from build123d import *

# Parameters (mm, degrees)
F0_R      = 2.05
F1_DEPTH  = 0.8
F2_DEPTH  = 19.2
F3_R      = 4.55
F4_DEPTH  = 2.1
F5_DEPTH  = 4
F6_DEPTH  = 10.3
F8_W      = 14.5
F8_H      = 16.5
F12_DEPTH = 0.65
F13_R     = 2.1
F14_SIZE  = 0.2


with BuildPart() as f1:
    # F0 (on Top) → F1 (new body)
    with BuildSketch(Plane.XY):
        with BuildLine():
            ThreePointArc((-13.5296202829, -3.5), (-13.975, 0), (-13.5296202829, 3.5))
            Line((-13.5296202829, 3.5), (-17.45, 3.5))
            ThreePointArc((-17.45, 3.5), (-20.95, 0), (-17.45, -3.5))
            Line((-17.45, -3.5), (-13.5296202829, -3.5))
        make_face()
        with Locations((-17.45, 0)):
            Circle(F0_R, mode=Mode.SUBTRACT)
    extrude(amount=F1_DEPTH)



with BuildPart() as f1b:
    # F0 (on Top) → F1, piece 2 (new body)
    with BuildSketch(Plane.XY):
        with BuildLine():
            Line((17.45, 3.5), (13.5296202829, 3.5))
            ThreePointArc((13.5296202829, 3.5), (13.975, 0), (13.5296202829, -3.5))
            Line((13.5296202829, -3.5), (17.45, -3.5))
            ThreePointArc((17.45, -3.5), (20.95, 0), (17.45, 3.5))
        make_face()
        with Locations((17.45, 0)):
            Circle(F0_R, mode=Mode.SUBTRACT)
    extrude(amount=F1_DEPTH)


with BuildPart() as f1_1:
    add(f1.part)

    add(f1b.part)  # F2 merges F1b
    # F0 (on Top) → F2 (join)
    with BuildSketch(Plane.XY):
        with BuildLine():
            ThreePointArc((13.5296202829, -3.5), (13.975, 0), (13.5296202829, 3.5))
            ThreePointArc((13.5296202829, 3.5), (0, 13.975), (-13.5296202829, 3.5))
            ThreePointArc((-13.5296202829, 3.5), (-13.975, 0), (-13.5296202829, -3.5))
            ThreePointArc((-13.5296202829, -3.5), (0, -13.975), (13.5296202829, -3.5))
        make_face()
    extrude(amount=F2_DEPTH)

    # F3 (on Top) → F4 (join)
    with BuildSketch(Plane.XY):
        with Locations((0, -7.825)):
            Circle(F3_R)
        with BuildLine():
            ThreePointArc((1.475, -5.8687599841), (2.1927437151, -6.7321253503), (2.45, -7.825))
            ThreePointArc((2.45, -7.825), (2.1927437151, -8.9178746497), (1.475, -9.7812400159))
            ThreePointArc((1.475, -9.7812400159), (0, -10.275), (-1.475, -9.7812400159))
            ThreePointArc((-1.475, -9.7812400159), (-2.45, -7.825), (-1.475, -5.8687599841))
            ThreePointArc((-1.475, -5.8687599841), (0, -5.375), (1.475, -5.8687599841))
        make_face(mode=Mode.SUBTRACT)
    extrude(amount=-F4_DEPTH)

    # F3 (on Top) → F5 (join)
    with BuildSketch(Plane.XY):
        with BuildLine():
            ThreePointArc((1.475, -9.7812400159), (2.1927437151, -8.9178746497), (2.45, -7.825))
            ThreePointArc((2.45, -7.825), (2.1927437151, -6.7321253503), (1.475, -5.8687599841))
            Line((1.475, -5.8687599841), (1.475, -9.7812400159))
        make_face()
        with BuildLine():
            Line((1.475, -9.7812400159), (1.475, -5.8687599841))
            ThreePointArc((1.475, -5.8687599841), (0, -5.375), (-1.475, -5.8687599841))
            Line((-1.475, -5.8687599841), (-1.475, -9.7812400159))
            ThreePointArc((-1.475, -9.7812400159), (0, -10.275), (1.475, -9.7812400159))
        make_face()
        with BuildLine():
            Line((-1.475, -9.7812400159), (-1.475, -5.8687599841))
            ThreePointArc((-1.475, -5.8687599841), (-2.45, -7.825), (-1.475, -9.7812400159))
        make_face()
    extrude(amount=-F5_DEPTH)

    # F3 (on Top) → F6 (join)
    with BuildSketch(Plane.XY):
        with BuildLine():
            Line((1.475, -9.7812400159), (1.475, -5.8687599841))
            ThreePointArc((1.475, -5.8687599841), (0, -5.375), (-1.475, -5.8687599841))
            Line((-1.475, -5.8687599841), (-1.475, -9.7812400159))
            ThreePointArc((-1.475, -9.7812400159), (0, -10.275), (1.475, -9.7812400159))
        make_face()
    extrude(amount=-F6_DEPTH)

    # F8 (on offset) → F9 (join, up to the next surface of F1)
    with BuildSketch(Plane.XZ.offset(-17.175)):
        with Locations((0, 8.25)):
            Rectangle(F8_W, F8_H)
    extrude(until=Until.NEXT)

    # F11 (on offset) → F12 (cut, through all)
    with BuildSketch(Plane.XY.offset(17.15)):
        with BuildLine():
            Line((-8.625, 12.9959083299), (-8.625, 11.5))
            ThreePointArc((-8.625, 11.5), (-7.9506110955, 11.9761599943), (-7.25, 12.4128209928))
            Line((-7.25, 12.4128209928), (-7.25, 13.8205759578))
            ThreePointArc((-7.25, 13.8205759578), (-7.9482026537, 13.4260870893), (-8.625, 12.9959083299))
        make_face()
        with BuildLine():
            ThreePointArc((7.25, 12.4128209928), (7.9506110955, 11.9761599943), (8.625, 11.5))
            Line((8.625, 11.5), (8.625, 12.9959083299))
            ThreePointArc((8.625, 12.9959083299), (7.9482026537, 13.4260870893), (7.25, 13.8205759578))
            Line((7.25, 13.8205759578), (7.25, 12.4128209928))
        make_face()
    extrude(amount=-F12_DEPTH, mode=Mode.SUBTRACT)

    # F13
    f13_edges = [f1_1.edges().sort_by_distance(p)[0] for p in [
        (-13.52962, -3.5, 19.2),
    ]]
    fillet(f13_edges, radius=F13_R)

    # F14
    f14_edges = [f1_1.edges().sort_by_distance(p)[0] for p in [
        (0, -5.375, -10.3),
        (0, -10.275, -10.3),
    ]]
    chamfer(f14_edges, length=F14_SIZE)


solid = f1_1.part
Can you work these out from the model? Positions are in its coordinate system, mm. A direction names the side the tool comes from. Coordinates: 2 decimals unless noted, no trailing zeros. Write each loop counter-clockwise with the first axis right and the second up, starting at its lowest first coordinate (ties: lowest second). Pieces come first, ordered by that corner, then holes.
Q1. Which directions (+Z, -Z, +X, -X, +Y, -Y) give clear straight access to the entire face, cutting with the end or side of a thin tool? Please do faces 1 (the face through (2, -8, -4)), 2 (the face through (4.34, -6.46, -1.04)), 3 (the face through (7.25, 15, 8)).
Results found:
face 1: -Z, +X, +Y, -Y
face 2: -Z
face 3: +Z, -Z, +X, +Y
Q2. For P1, Ø6.5, axis at x = 17.45, y = 0, coming from the +Z side; P2, Ø2, axis at y = -4.5, z = -2, coming from the -X side; P3, Ø2, axis at x = -12.5, z = 3.5, coming from the -Y side, each with a flat end and sliding along its axis, tell me the tip position at first contact or that it passes through.
Results found:
P1: stops at z = 0.8
P2: stops at x = -3.91
P3: stops at y = -7.94
Q3. Imagine slicing it at C-C, the plane z = 5. List the corners of the cut face in (x, y) for me (3 decimals), plus the area to 3 significant figures.
Results found:
outline: (-7.25, 11.947) arc R13.975 ccw (long way) to (7.25, 11.947) - (7.25, 17.175) - (-7.25, 17.175) - close
area: 669 mm2
Q4. Imagine slicing it at D-D, the plane y = 15. List the corners of the cut face in (x, z) for me, plus the area to 3 significant figures.
Results found:
outline: (-7.25, 0) - (7.25, 0) - (7.25, 16.5) - (-7.25, 16.5) - close
area: 239 mm2
Q5. Imagine slicing it at B-B, the plane x = 0. List the corners of the cut face in (y, z) for me (3 decimals).
Results found:
outline: (-13.975, 0) - (-12.375, 0) - (-12.375, -2.1) - (-10.275, -2.1) - (-10.275, -10.1) - (-10.075, -10.3) - (-5.575, -10.3) - (-5.375, -10.1) - (-5.375, -2.1) - (-3.275, -2.1) - (-3.275, 0) - (17.175, 0) - (17.175, 16.5) - (13.975, 16.5) - (13.975, 17.1) arc R2.1 ccw to (11.875, 19.2) - (-11.875, 19.2) arc R2.1 ccw to (-13.975, 17.1) - close
Q6. Imagine slicing it at A-A, the plane y = 0. List the corners of the cut face in (x, z) for me (3 decimals), plus the area to 3 significant figures.
Results found:
outline: (-20.95, 0) - (-19.5, 0) - (-19.5, 0.8) - (-20.95, 0.8) - close; (-15.4, 0) - (15.4, 0) - (15.4, 0.8) - (13.975, 0.8) - (13.975, 17.1) arc R2.1 ccw to (11.875, 19.2) - (-11.875, 19.2) arc R2.1 ccw to (-13.975, 17.1) - (-13.975, 0.8) - (-15.4, 0.8) - close; (19.5, 0) - (20.95, 0) - (20.95, 0.8) - (19.5, 0.8) - close
area: 539 mm2
Q7. Please list where these lines run through material, in increasing order: L1, parallel to Y at x = -17.45, z = 0.6; L2, parallel to Z at x = 3, y = 1.5; L3, parallel to Z at x = 1, y = -3.5.
Results found:
L1: y = -3.5 to -2.05, 2.05 to 3.5
L2: z = 0 to 19.2
L3: z = -2.1 to 19.2
Q8. If we mould it in two halves opening along X, with no side actions, what happens to faces 4 (the face through (-1.475, -8, -7)), 5 (the face through (-19.5, 0.09, 0.39)), 6 (the face through (-2, -8, -4))? For each: +X half, -X half, draft (parallel to the pull), parting line (faces both ways), or undercut.
Results found:
face 4: -X half
face 5: undercut
face 6: draft
